```python
from build123d import *

# Parameters (mm, degrees)
SKETCH2_R                = 7.5
BOSS_EXTRUDE1_DEPTH      = 109
BOSS_EXTRUDE1_DEPTH_BACK = 15
SKETCH4_W                = 50
SKETCH4_H                = 50
BOSS_EXTRUDE2_DEPTH      = 20


with BuildPart() as part:
    # Sketch1 → Revolve1 (revolve)
    with BuildSketch(Plane.XY):
        Polygon((0, 50), (25, 50), (25.25, 49), (0, 49), align=None)
        Polygon((50, -50), (0, -50), (0, -49), (49.75, -49), align=None)
        Polygon((0, -39), (47.25, -39), (47.5, -40), (0, -40), align=None)
        Polygon((0, -29), (44.75, -29), (45, -30), (0, -30), align=None)
        Polygon((0, -19), (42.25, -19), (42.5, -20), (0, -20), align=None)
        Polygon((0, -9), (39.75, -9), (40, -10), (0, -10), align=None)
        Polygon((0, 1), (37.25, 1), (37.5, 0), (0, 0), align=None)
        Polygon((0, 11), (34.75, 11), (35, 10), (0, 10), align=None)
        Polygon((0, 21), (32.25, 21), (32.5, 20), (0, 20), align=None)
        Polygon((0, 31), (29.75, 31), (30, 30), (0, 30), align=None)
        Polygon((0, 41), (27.25, 41), (27.5, 40), (0, 40), align=None)
    revolve(axis=Axis((0, -50, 0), (0, 1, 0)))

    # Sketch2 → Boss-Extrude1 (add, two sides)
    with BuildSketch(Plane(origin=(0, -49, 0), x_dir=(1, 0, 0), z_dir=(0, 1, 0))) as boss_extrude1_sk:
        Circle(SKETCH2_R)
    extrude(amount=BOSS_EXTRUDE1_DEPTH)
    extrude(boss_extrude1_sk.sketch, amount=-BOSS_EXTRUDE1_DEPTH_BACK)

    # Sketch3 → Revolve2 (revolve)
    with BuildSketch(Plane.XY):
        with BuildLine():
            Line((0, 85), (0, 55))
            ThreePointArc((0, 55), (15, 70), (0, 85))
        make_face()
    revolve(axis=Axis((0, -55, 0), (0, 1, 0)))

    # Sketch4 → Boss-Extrude2 (add)
    with BuildSketch(Plane.XZ.offset(64)):
        Rectangle(SKETCH4_W, SKETCH4_H)
    extrude(amount=BOSS_EXTRUDE2_DEPTH)


solid = part.part
```
Verification items for the finished model (mm, model axes). A direction names the side the tool comes from. Give positions to 0.01 mm unless a question says otherwise; leave off trailing zeros. Order: outer loops, then holes, each group sorted by start corner. A loop starts at its lowest first (then second) coordinate and runs counter-clockwise, first axis right, second up. Notation, with made-up numbers: (84.5, 63) -> (99.5, 63) arc R20 cw to (99.5, 70) -> close; hole circle Ø7 at (6, 64.5). An arc over 180 degrees is marked (long way). Use a Markdown table: item, result.
1) Depth check by flat-ended pin: pin 1 Ø16 at (x, y) = (4, -72.5) entering from +Z; pin 2 Ø1.5 at (x, z) = (2.5, 38.5) entering from +Y; pin 3 Ø8 at (x, y) = (22, 31) entering from +Z; pin 4 Ø2 at (y, z) = (22.5, 32.5) entering from -X. Enter the tip coordinate at first touch or a pass-through.
Results:
| item | result |
|---|---|
| pin 1 | z = 25 |
| pin 2 | y = -9 |
| pin 3 | z = 23.9 |
| pin 4 | through |
2) Tool access check on faces 1 (the flat face through (-25, -74, 0)), 2 (the flat face through (25, -74, 0)), 3 (the flat face through (-6, -64, 6)). Record the directions out of +Z, -Z, +X, -X, +Y, -Y that give a thin tool (end or side, any length) a straight path to the whole face; none if there is none.
Results:
| item | result |
|---|---|
| face 1 | +Z, -Z, -X, -Y |
| face 2 | +Z, -Z, +X, -Y |
| face 3 | none |
3) Section check C-C, the plane y = 25. Record the boundary of the cut face in (x, z), then the cut area to 3 significant figures.
Results:
| item | result |
|---|---|
| outline | circle Ø15 at (0, 0) |
| area | 177 mm² |
4) Material ranges on probe 1 along Y at (x, z) = (-33.5, -16); probe 2 along Y at (x, z) = (-13, 39); probe 3 along Y at (x, z) = (-40, -20), recorded low to high.
Results:
| item | result |
|---|---|
| probe 1 | -50 to -49, -40 to -39, -30 to -29, -20 to -19, -10 to -9, 0 to 1 |
| probe 2 | -50 to -49, -40 to -39, -30 to -29, -20 to -19 |
| probe 3 | -50 to -49, -40 to -39, -30 to -29 |
5) Section check A-A, the plane x = 20.5. Give the number of separate pieces and of enclosed holes in the cut face, then the cut area to 3 significant figures.
Results:
| item | result |
|---|---|
| separate pieces | 12 |
| enclosed holes | 0 |
| area | 1,680 mm² |
